Part print with two shaded views. Sizes in mm from the minimum x, y, z corner. A direction names the side the tool comes from. Round coordinates to 2 decimals unless told otherwise and drop trailing zeros. Write each loop counter-clockwise with the first axis right and the second up, starting at its lowest first coordinate (ties: lowest second). Pieces come first, ordered by that corner, then holes. Notation, with made-up numbers: M -3.5,76.5 L 52.5,76.5 A22 cw 52.5,108.5 Z; hole C -19,-26 d8. An arc over 180 degrees is marked long. Use one line per item in the form item = value. Start each with the question number.
Item 1: Cut at A-A, the plane z = 11. Give the cut face in (x, y).
Item 2: Flat gauge pins, fed straight in: pin 1 Ø1 at (x, y) = (16.5, 2) entering from +Z; pin 2 Ø1.5 at (y, z) = (1, 13.5) entering from +X. Where does each tip first touch, or does it go through?
Item 3: Cut at C-C, the plane y = 3.5. Give the cut face in (x, z), then the cut area to 3 significant figures.
Item 4: Probe L1, parallel to Z at x = 11, y = 3.3; L2, parallel to Z at x = 11, y = 2.5; L3, parallel to X at y = 2.25, z = 14.25. List the from-to ranges inside material, lowest first.
Item 5: Mould opens along Z. For the marked faces 1, 2 and 3 say: +Z half, -Z half, draft (parallel to the pull), parting line (faces both ways), or undercut.
Item 6: Cut at D-D, the plane y = 1.2. Give the cut face in (x, z), then the cut area to 3 significant figures.
Item 7: Cut at B-B, the plane x = 11. Give the cut face in (y, z), then the cut area to 4 significant figures.
Item 8: Which spindle directions (+Z, -Z, +X, -X, +Y, -Y) get a long thin tool onto all of the face, cutting with end or side? Do the marked faces 4 and 5. Say none if no direction does.
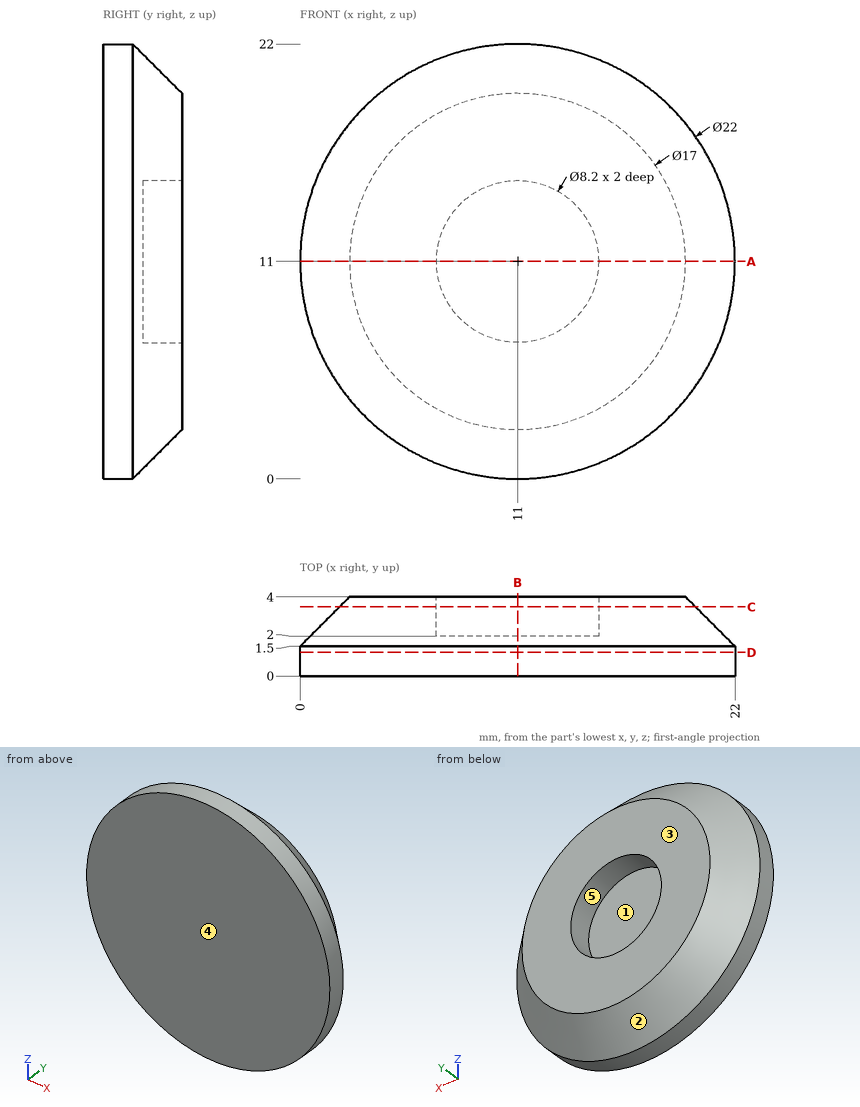
Model answer:
q1.outline = M 0,0 L 22,0 L 22,1.5 L 19.5,4 L 15.1,4 L 15.1,2 L 6.9,2 L 6.9,4 L 2.5,4 L 0,1.5 Z
q2.pin_1 = 20.59
q2.pin_2 = 21.86
q3.outline = C 11,11 d18; hole C 11,11 d8.2
q3.area = 202 mm²
q4.L1 = 1.8 to 6.9, 15.1 to 20.2
q4.L2 = 1 to 6.9, 15.1 to 21
q4.L3 = 1.28 to 8.5, 13.5 to 20.72
q5.face_1 = undercut
q5.face_2 = parting line
q5.face_3 = draft
q6.outline = C 11,11 d22
q6.area = 380 mm²
q7.outline = M 0,0 L 1.5,0 L 4,2.5 L 4,6.9 L 2,6.9 L 2,15.1 L 4,15.1 L 4,19.5 L 1.5,22 L 0,22 Z
q7.area = 65.35 mm²
q8.face_4 = +Z, -Z, +X, -X, -Y
q8.face_5 = +Y
